from build123d import *

# Parameters (mm, degrees)
SKETCH_1_R      = 1.6
EXTRUDE_1_DEPTH = 2


with BuildPart() as part:
    # 草图1 → 凸台-拉伸1 (new body)
    with BuildSketch(Plane(origin=(0, 0, 0), x_dir=(1, 0, 0), z_dir=(0, 1, 0))):
        with BuildLine():
            Line((0, -4), (-33.5, -4))
            ThreePointArc((-33.5, -4), (-37.5, 0), (-33.5, 4))
            Line((-33.5, 4), (0, 4))
            ThreePointArc((0, 4), (4, 0), (0, -4))
        make_face()
        Circle(SKETCH_1_R, mode=Mode.SUBTRACT)
        with BuildLine():
            Line((-33.5, 1.6), (-7.5, 1.6))
            ThreePointArc((-7.5, 1.6), (-5.9, 0), (-7.5, -1.6))
            Line((-7.5, -1.6), (-33.5, -1.6))
            ThreePointArc((-33.5, -1.6), (-35.1, 0), (-33.5, 1.6))
        make_face(mode=Mode.SUBTRACT)
    extrude(amount=EXTRUDE_1_DEPTH)


solid = part.part
Read the model definition and answer for the solid it produces. Units are mm, in the model's axes. A direction names the side the tool comes from. Round coordinates to 2 decimals unless told otherwise and drop trailing zeros. Write each loop counter-clockwise with the first axis right and the second up, starting at its lowest first coordinate (ties: lowest second). Pieces come first, ordered by that corner, then holes. Notation, with made-up numbers: M -0.5,49 L 13.5,49 A21 ccw 13.5,63 Z; hole C 84,75.5 d7. An arc over 180 degrees is marked long. Use a Markdown table: item, result.
1) A tool of negligible diameter and unlimited length cuts with its end or side. For faces 1 (the cylindrical face through (-5.9, 1, 0)), 2 (the flat face through (-17, 1, -4)), from which of +Z, -Z, +X, -X, +Y, -Y can it reach the whole face along a straight path? Write none if from no direction.
Answers follow:
| item | result |
|---|---|
| face 1 | +Y, -Y |
| face 2 | -Z, +X, -X, +Y, -Y |
2) The part is cut by section D-D (z = 3). Write down the section's boundary in (x, y), plus the area to 3 significant figures.
Answers follow:
| item | result |
|---|---|
| outline | M -36.15,0 L 2.65,0 L 2.65,2 L -36.15,2 Z |
| area | 77.6 mm2 |
3) The part is cut by section A-A (y = 0.65). Write down the section's boundary in (x, z).
Answers follow:
| item | result |
|---|---|
| outline | M -33.5,-4 L 0,-4 A4 ccw 0,4 L -33.5,4 A4 ccw Z; hole M -33.5,-1.6 L -7.5,-1.6 A1.6 ccw -7.5,1.6 L -33.5,1.6 A1.6 ccw Z; hole C 0,0 d3.2 |
4) The part is cut by section C-C (z = 0). Write down the section's boundary in (x, y), plus the area to 3 significant figures.
Answers follow:
| item | result |
|---|---|
| outline | M -37.5,0 L -35.1,0 L -35.1,2 L -37.5,2 Z; M -5.9,0 L -1.6,0 L -1.6,2 L -5.9,2 Z; M 1.6,0 L 4,0 L 4,2 L 1.6,2 Z |
| area | 18.2 mm2 |
5) Straight lines are drawn through the part: line 1 along X through (y, z) = (1.35, 0); line 2 along Z through (x, y) = (-29, 1.2); line 3 along Z through (x, y) = (-1, 1.6). For each, find the intervals that lie inside material, in ascending order. Write a range as [from, to].
Answers follow:
| item | result |
|---|---|
| line 1 | x = [-37.5, -35.1], [-5.9, -1.6], [1.6, 4] |
| line 2 | z = [-4, -1.6], [1.6, 4] |
| line 3 | z = [-4, -1.25], [1.25, 4] |
6) The part is cut by section B-B (x = -25.5). Write down the section's boundary in (y, z).
Answers follow:
| item | result |
|---|---|
| outline | M 0,-4 L 2,-4 L 2,-1.6 L 0,-1.6 Z; M 0,1.6 L 2,1.6 L 2,4 L 0,4 Z |
7) For a pull along X with two mould halves and no side action, classify faces 3 (the flat face through (-21, 1, -1.6)), 4 (the flat face through (-16, 0, -2)), 5 (the cylindrical face through (-37.5, 1, 0.1)) as pulls with the +X half, pulls with the -X half, needs draft (parallel to the pull), parting line crosses it, or undercut.
Answers follow:
| item | result |
|---|---|
| face 3 | undercut |
| face 4 | needs draft |
| face 5 | pulls with the -X half |
